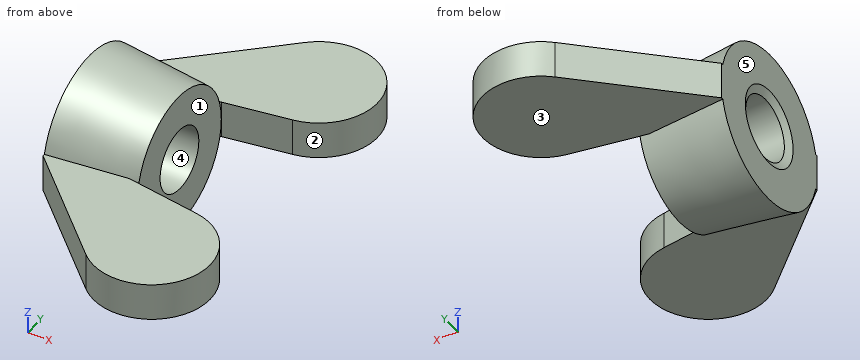
Autodesk Inventor part; units mm, degrees
ref_plane "Work Plane1" through (23.9635, 0, 0) normal (0, 0, -1) x (1, 0, 0)
ref_plane "YZ Plane" through (0, 0, 0) normal (1, 0, 0) x (0, 1, 0)
ref_plane "XZ Plane" through (0, 0, 0) normal (0, 1, 0) x (-1, 0, 0)
sketch "Sketch1" plane through (0, 0, 0) normal (0, 0, 1) x (1, 0, 0)
  line L0 (0, 0) -> (4.6, 0)
  line L1 (0, 0) -> (0, 4)
  line L2 (4.6, 3.5) -> (4.6, 0)
  line L3 (0, 4) -> (5.431, 9.1724)
  line L4 (4.6, 3.5) -> (7.9721, 4.0374)
  arc A0 (7.9721, 4.0374) -> (5.431, 9.1724) centre (7.5, 7) ccw
  line L5 (4.6, 3.5) -> (0, 4)
  line L6 (4.6, 3.5) -> (0, 2.7669)
  dimension "d0" = 7
  dimension "d1" = 7.5
  dimension "d2" = 7
  dimension "d3" = 3
  dimension "d4" = 4.6
  dimension "d5" = 8
revolve "Body" add sketch "Sketch1" angle 360 about axis through (0, 0, 0) along (1, 0, 0) contours L1 L6 L2 L0 | L1 L5 L6
extrude "Wing1" add sketch "Sketch1" along normal mid plane 1.9 contours L1 L5 L6 | L5 L3 A0 L4
fillet "Fillet1" [suppressed]
mirror "Wing2" about plane through (0, 0, 0) normal (0, 1, 0) of "Wing1"
sketch "Sketch2" plane through (0, 0, 0) normal (1, 0, 0) x (0, 1, 0)
  line L0 (0, -14) -> (0, 14)
  line L1 (-14, 0) -> (14, 0)
  point P0 (0, 0)
hole "Thread" at (0, 0, 0) direction (1, 0, 0) diameter 3.242 end through all
chamfer "Chamfer1" distance 0.3789 angle 30 1 edges at (0, 0, -1.621) measured on face at (0, -3.1268, -0.0651)
ref_plane "Work Plane1" through (23.9635, 0, 0) normal (0, 0, -1) x (1, 0, 0)
equation "\"d0\" = KOD2"
equation "\"d1\" = KOH1 - RR"
equation "\"d2\" = 0.5 * E0 - RR"
equation "\"d3\" = RR"
equation "\"d4\" = KOH"
equation "\"d5\" = KOD"
equation "\"d6\" = SW"
equation "\"d8\" = 0.333333 * SW"
equation "\"d9\" = -0.5 * GD1 + 0.5 * NND"
equation "\"d109\" = -0.5 * GD1 + 0.5 * NND"
equation "\"NND\" = 4"
equation "\"KOH\" = 4.6"
equation "\"KOH1\" = 10.5"
equation "\"SW\" = 1.9"
equation "\"KOD\" = 8"
equation "\"KOD2\" = 7"
equation "\"RR\" = 3"
equation "\"GUL\" = 0.541266 * PTC"
equation "\"BOR\" = 0"
equation "\"PTC\" = 0.7"
equation "\"THREADDIA\" = 4"
equation "\"TOA\" = 30deg"
equation "\"RR2\" = 2"
equation "\"SW1\" = 2.3"
equation "\"GAL\" = 0.541266 * PTC"
properties part number "DIN 315 - M4" material "Steel, Mild"
Geometry check sheet. Reference: the model listing, model coordinates, mm. Face numbers are marked on the shaded views. A direction names the side the tool comes from. Give positions to 0.01 mm unless a question says otherwise; leave off trailing zeros. Order: outer loops, then holes, each group sorted by start corner. A loop starts at its lowest first (then second) coordinate and runs counter-clockwise, first axis right, second up. Notation, with made-up numbers: (77.25, -4) - (106.25, -4) arc R25 ccw to (106.25, 10) - close; hole circle Ø5 at (80, 22.25). An arc over 180 degrees is marked (long way). Answer as a JSON object with one key per item and string values.
(1) Cross-section at B-B (x = 3.25). Record the cut outline in (y, z), then the cut area to 3 significant figures.
Report:
{"outline": "(-7.1, -0.95) - (-3.52, -0.95) arc R3.65 ccw to (3.52, -0.95) - (7.1, -0.95) - (7.1, 0.95) - (3.52, 0.95) arc R3.65 ccw to (-3.52, 0.95) - (-7.1, 0.95) - close; hole circle Ø3.24 at (0, 0)", "area": "46.8 mm^2"}
(2) Cross-section at C-C (x = 7.5). Record the cut outline in (y, z).
Report:
{"outline": "(-10, -0.95) - (-3.96, -0.95) - (-3.96, 0.95) - (-10, 0.95) - close; (3.96, -0.95) - (10, -0.95) - (10, 0.95) - (3.96, 0.95) - close"}
(3) Depth check by flat-ended pin: pin 1 Ø2 at (x, y) = (6.5, 7) entering from -Z; pin 2 Ø4 at (x, y) = (2.5, 0.5) entering from +Z; pin 3 Ø4 at (x, z) = (6, -2) entering from -Y; pin 4 Ø3.5 at (x, y) = (4, -5.5) entering from +Z. Enter the tip coordinate at first touch or a pass-through.
Report:
{"pin 1": "z = -0.95", "pin 2": "z = 3.94", "pin 3": "y = -10", "pin 4": "z = 0.95"}
(4) Tool access check on the marked faces 1 and 2. Record the directions out of +Z, -Z, +X, -X, +Y, -Y that give a thin tool (end or side, any length) a straight path to the whole face; none if there is none.
Report:
{"face 1": "+Z, -Z, +X", "face 2": "+Z, -Z"}
(5) Draft check along Z on the marked faces 3, 4 and 5. Enter one of: released by +Z, released by -Z, zero draft, split by the parting line, or undercut.
Report:
{"face 3": "released by -Z", "face 4": "undercut", "face 5": "zero draft"}
(6) Cross-section at D-D (y = 8.75). Record the cut outline in (x, z).
Report:
{"outline": "(4.99, -0.95) - (9.94, -0.95) - (9.94, 0.95) - (4.99, 0.95) - close"}
(7) Material ranges on line 1 (X direction, y = -1.5, z = -1.75); line 2 (Z direction, x = 1.65, y = 0); line 3 (Z direction, x = 9.25, y = -8), recorded low to high.
Report:
{"line 1": "0 to 4.6", "line 2": "-3.82 to -1.62, 1.62 to 3.82", "line 3": "-0.95 to 0.95"}
(8) Cross-section at A-A (y = 0). Record the cut outline in (x, z).
Report:
{"outline": "(0, -4) - (4.6, -3.5) - (4.6, -1.62) - (0.22, -1.62) - (0, -2) - close; (0, 2) - (0.22, 1.62) - (4.6, 1.62) - (4.6, 3.5) - (0, 4) - close"}
